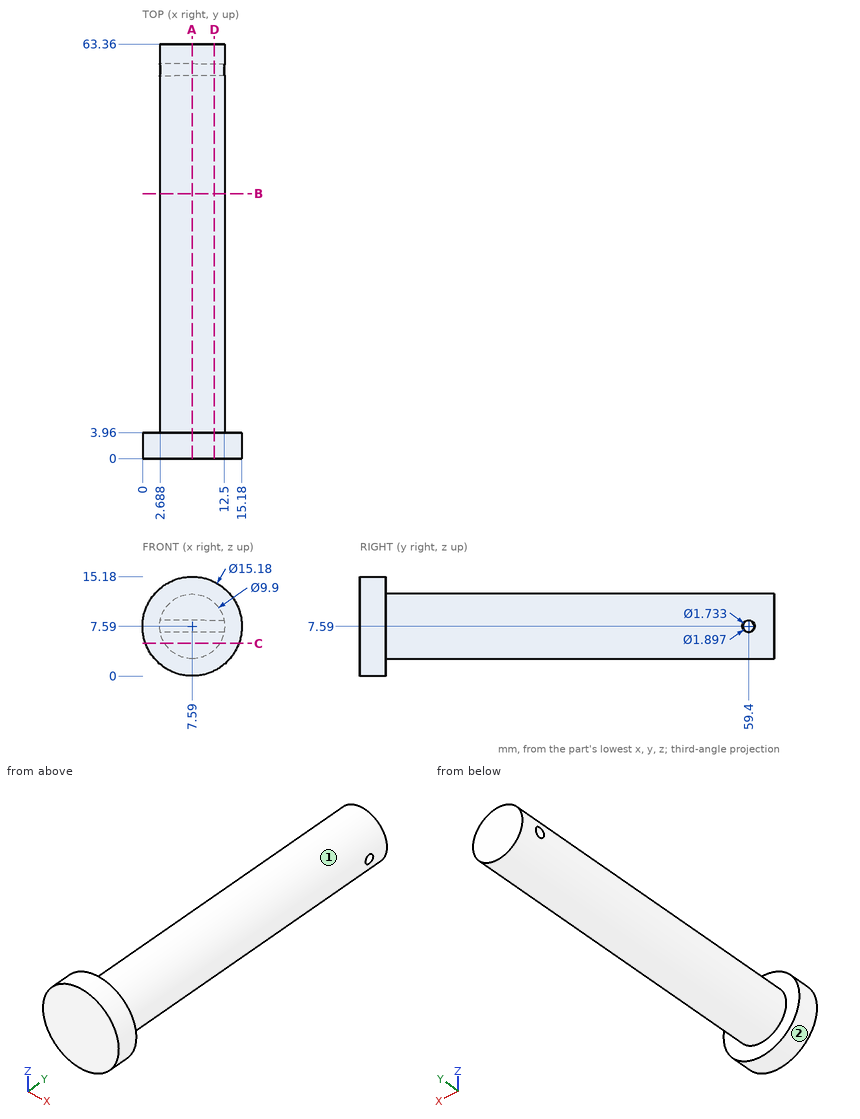
Here's the drawing with two shaded views (mm, measured from the low corner). I have some questions. A direction names the side the tool comes from. Coordinates: 2 decimals unless noted, no trailing zeros. Order: outer loops, then holes, each group sorted by start corner. A loop starts at its lowest first (then second) coordinate and runs counter-clockwise, first axis right, second up. Notation, with made-up numbers: (16.25, -35.75) - (31.25, -35.75) arc R32 cw to (31.25, -2.75) - close; hole circle Ø7 at (-22, 71.5). An arc over 180 degrees is marked (long way). Answer in a Markdown table with one row per item. Add a question column.
(1) If we section it at C-C, the plane z = 5: Please give me the cut outline in (x, y) (1 decimal).
(2) If we section it at A-A, the plane x = 7.59: Please give me the cut outline in (y, z) (1 decimal).
(3) Will these pins go through, and if not, where does the flat tip stop? pin 1 (1 mm diameter, centred on x = 2.5, y = 50, fed in from -Z) (1 decimal); pin 2 (5 mm diameter, centred on x = 3, z = 4, fed in from +Y).
(4) I need wall thicknesses on L1, parallel to Y at x = 11, z = 13.75; L2, parallel to X at y = 60.5, z = 7.5; L3, parallel to Z at x = 8.5, y = 19 (1 decimal). Which ranges of each line are inside material? Lowest first, please.
(5) If we section it at B-B, the plane y = 40.5: Please give me the cut outline in (x, z).
(6) If we section it at D-D, the plane x = 11: Please give me the cut outline in (y, z).
(7) On a 3-axis mill with a long thin cutter (end or side, diameter ignored), from which of +Z, -Z, +X, -X, +Y, -Y can I reach the whole of each face in a straight line? I mean the marked faces 1 and 2. Say none if no direction works.
Results are:
| question | item | result |
|---|---|---|
| 1 | outline | (0.5, 0) - (14.7, 0) - (14.7, 4) - (11.8, 4) - (11.8, 63.4) - (3.4, 63.4) - (3.4, 4) - (0.5, 4) - close |
| 2 | outline | (0, 0) - (4, 0) - (4, 2.6) - (63.4, 2.6) - (63.4, 12.5) - (4, 12.5) - (4, 15.2) - (0, 15.2) - close; hole circle Ø1.8 at (59.4, 7.6) |
| 3 | pin 1 | stops at z = 5.7 |
| 3 | pin 2 | stops at y = 63.36 |
| 4 | L1 | y = 0 to 3.96 |
| 4 | L2 | x = 2.64 to 12.54 |
| 4 | L3 | z = 2.7 to 12.5 |
| 5 | outline | circle Ø9.9 at (7.59, 7.59) |
| 6 | outline | (0, 0.81) - (3.96, 0.81) - (3.96, 4) - (63.36, 4) - (63.36, 11.18) - (3.96, 11.18) - (3.96, 14.37) - (0, 14.37) - close; hole circle Ø1.76 at (59.4, 7.59) |
| 7 | face 1 | +Y |
| 7 | face 2 | +Y, -Y |
